```python
from build123d import *

# Parameters (mm, degrees)
F0_W     = 150
F0_H     = 220
F1_DEPTH = 8
F2_R     = 3
F2_R_2   = 4
F3_DEPTH = 12


with BuildPart() as f1:
    # F0 (on Front) → F1 (new body)
    with BuildSketch(Plane.XZ):
        with Locations((-75, -110)):
            Rectangle(F0_W, F0_H)
    extrude(amount=F1_DEPTH)

    # F2 (on face) → F3 (join)
    with BuildSketch(Plane.XZ.offset(8)):
        with Locations((-75, -187)):
            Circle(F2_R)
        with Locations((-35, -135)):
            Circle(F2_R_2)
        with Locations((-35, -160)):
            Circle(F2_R_2)
        with Locations((-115, -135)):
            Circle(F2_R_2)
        with Locations((-115, -160)):
            Circle(F2_R_2)
    extrude(amount=-F3_DEPTH)


solid = f1.part
```
Geometry check sheet. Reference: the model listing, model coordinates, mm. A direction names the side the tool comes from. Give positions to 0.01 mm unless a question says otherwise; leave off trailing zeros. Write each loop counter-clockwise with the first axis right and the second up, starting at its lowest first coordinate (ties: lowest second). Pieces come first, ordered by that corner, then holes.
1) Section check A-A, the plane x = -75. Record the boundary of the cut face in (y, z), and give its area (3 significant figures).
2) Access from +Z, -Z, +X, -X, +Y, -Y to the whole of each face (thin tool, end or side, straight path). Record for faces 1 (the flat face through (-76, -4, -220)), 2 (the cylindrical face through (-35.521, 1.972, -131.034)).
3) Section check C-C, the plane x = -35. Record the boundary of the cut face in (y, z), and give its area (3 significant figures).
4) Gauge pin test, flat ends, axial feed: pin 1 (3 mm diameter, centred on y = -6.5, z = -159.5, fed in from +X); pin 2 (5 mm diameter, centred on x = -18.5, z = -39.5, fed in from +Y). Record the tip position at first contact, or that the pin passes through.
5) Section check D-D, the plane z = -169. Record the boundary of the cut face in (x, y), and give its area (3 significant figures).
6) Material ranges on L1, parallel to Y at x = -112, z = -210; L2, parallel to X at y = 3.5, z = -138, recorded low to high.
7) Release check for a two-part mould opening along Z. For faces 3 (the flat face through (-115, 4, -135)), 4 (the flat face through (-76, -4, 0)), 5 (the cylindrical face through (-112.85, 1.972, -156.627)), 6 (the cylindrical face through (-75, 2, -184)) record: pulls with the +Z half, pulls with the -Z half, needs draft (parallel to the pull), parting line crosses it, or undercut.
8) Section check B-B, the plane z = -135. Record the boundary of the cut face in (x, y).
Computed:
1. outline: (-8, -220) - (0, -220) - (0, -190) - (4, -190) - (4, -184) - (0, -184) - (0, 0) - (-8, 0) - close
1. area: 1,780 mm2
2. face 1: -Z, +X, -X, +Y, -Y
2. face 2: +Y
3. outline: (-8, -220) - (0, -220) - (0, -164) - (4, -164) - (4, -156) - (0, -156) - (0, -139) - (4, -139) - (4, -131) - (0, -131) - (0, 0) - (-8, 0) - close
3. area: 1,820 mm2
4. pin 1: stops at x = 0
4. pin 2: stops at y = 0
5. outline: (-150, -8) - (0, -8) - (0, 0) - (-150, 0) - close
5. area: 1,200 mm2
6. L1: y = -8 to 0
6. L2: x = -117.65 to -112.35, -37.65 to -32.35
7. face 3: needs draft
7. face 4: pulls with the +Z half
7. face 5: undercut
7. face 6: parting line crosses it
8. outline: (-150, -8) - (0, -8) - (0, 0) - (-31, 0) - (-31, 4) - (-39, 4) - (-39, 0) - (-111, 0) - (-111, 4) - (-119, 4) - (-119, 0) - (-150, 0) - close
